Source: three-view drawing plus pictorial views. Frame: mm from the lowest corner of the part. A direction names the side the tool comes from. Coordinates: 2 decimals unless noted, no trailing zeros. Order: outer loops, then holes, each group sorted by start corner. A loop starts at its lowest first (then second) coordinate and runs counter-clockwise, first axis right, second up. Notation, with made-up numbers: (-3, -30.75) -> (13, -30.75) arc R18 ccw to (13, -16.75) -> close; hole circle Ø5 at (3.25, 54). An arc over 180 degrees is marked (long way). One line per question, with ' | ' between items.
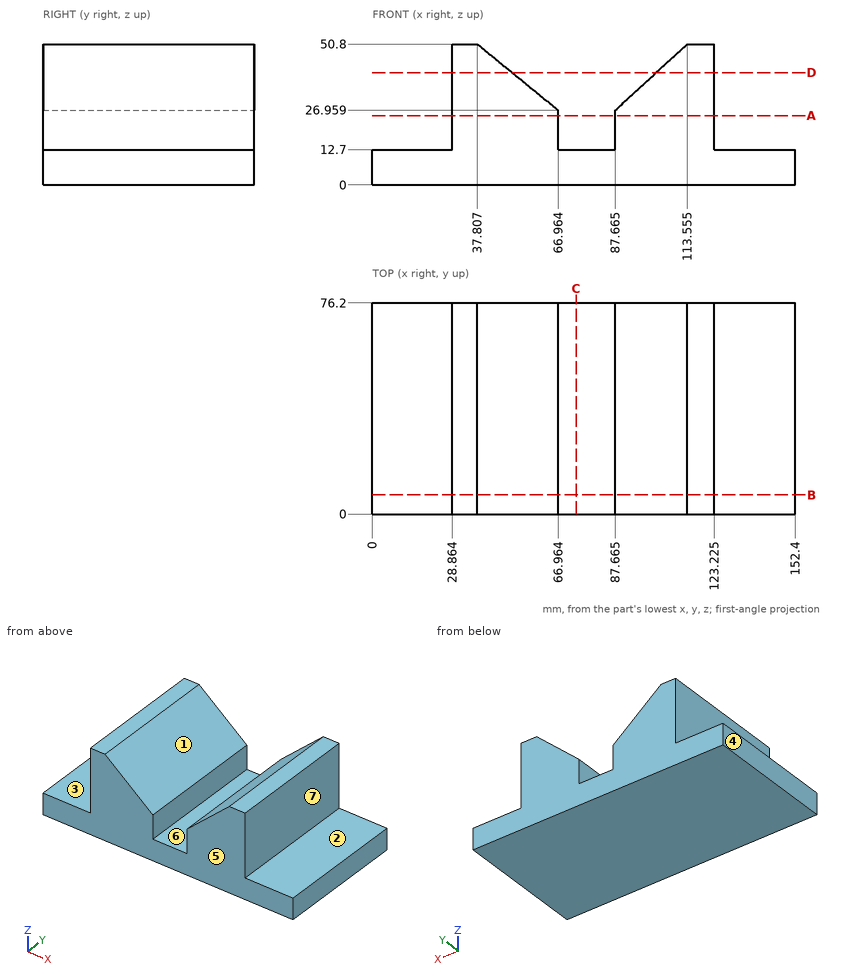
1. Cut plane C-C, the plane x = 73.5. Return loops of the section in (y, z).
Recorded:
outline: (0, 0) -> (76.2, 0) -> (76.2, 12.7) -> (0, 12.7) -> close
2. Cut plane D-D, the plane z = 40.5. Return loops of the section in (x, y) (1 decimal), and give its area (3 significant figures).
Recorded:
outline: (28.9, 0) -> (50.4, 0) -> (50.4, 76.2) -> (28.9, 76.2) -> close; (102.4, 0) -> (123.2, 0) -> (123.2, 76.2) -> (102.4, 76.2) -> close | area: 3,230 mm^2
3. Mould query, pull axis X, two halves, no side actions, for the marked faces 5, 6 and 7. Classes: released by +X, released by -X, zero draft, split by the parting line, or undercut.
Recorded:
face 5: zero draft | face 6: undercut | face 7: released by +X
4. Ray query, line 1 (X direction, y = 67, z = 24.5) (1 decimal); line 2 (Z direction, x = 127.5, y = 59.5); line 3 (X direction, y = 46.5, z = 37) (1 decimal). Return the intervals inside material, ascending. Write a range as [from, to].
Recorded:
line 1: x = [28.9, 67], [87.7, 123.2] | line 2: z = [0, 12.7] | line 3: x = [28.9, 54.7], [98.6, 123.2]
5. Access query for the marked faces 1, 2, 3 and 4. Directions: +Z, -Z, +X, -X, +Y, -Y. A direction counts if a zero-diameter tool reaches every point of the face in a straight line with its end or side. Return the directions, or none.
Recorded:
face 1: +Z, +Y, -Y | face 2: +Z, +X, +Y, -Y | face 3: +Z, -X, +Y, -Y | face 4: +Z, -Z, -X, +Y, -Y
6. Pin query (flat end, axial travel): pin 1 Ø16.5 at (x, y) = (80.5, 53.5) entering from +Z; pin 2 Ø6 at (x, y) = (75.5, 18.5) entering from +Z; pin 3 Ø4.5 at (y, z) = (21, 22.5) entering from +X (3 decimals). Return the tip coordinate at first contact, or that it passes through.
Recorded:
pin 1: stops at z = 27.96 | pin 2: stops at z = 12.7 | pin 3: stops at x = 123.225
7. Cut plane B-B, the plane y = 7. Return loops of the section in (x, z) (1 decimal), and give its area (3 significant figures).
Recorded:
outline: (0, 0) -> (152.4, 0) -> (152.4, 12.7) -> (123.2, 12.7) -> (123.2, 50.8) -> (113.6, 50.8) -> (87.7, 27) -> (87.7, 12.7) -> (67, 12.7) -> (67, 27) -> (37.8, 50.8) -> (28.9, 50.8) -> (28.9, 12.7) -> (0, 12.7) -> close | area: 4,090 mm^2
8. Cut plane A-A, the plane z = 25. Return loops of the section in (x, y) (1 decimal), and give its area (3 significant figures).
Recorded:
outline: (28.9, 0) -> (67, 0) -> (67, 76.2) -> (28.9, 76.2) -> close; (87.7, 0) -> (123.2, 0) -> (123.2, 76.2) -> (87.7, 76.2) -> close | area: 5,610 mm^2
